from build123d import *

# Parameters (mm, degrees)
F0_W     = 326.6186
F0_H     = 45.9232
F0_W_2   = 5.842
F0_H_2   = 12.7
F1_DEPTH = 5.842
F2_R     = 3.175
F3_R     = 2.0828
F4_DEPTH = 25.4
F5_R     = 2.0828
F6_DEPTH = 25.4
F7_W     = 12.7
F7_H     = 5.842
F7_R     = 1.7526
F8_DEPTH = 25.4


with BuildPart() as f1:
    # F0 (on Front) → F1 (new body)
    with BuildSketch(Plane.XZ):
        Rectangle(F0_W, F0_H)
        with Locations((-157.2133, -12.7)):
            Rectangle(F0_W_2, F0_H_2, mode=Mode.SUBTRACT)
        with Locations((-134.3787, -12.7)):
            Rectangle(F0_W_2, F0_H_2, mode=Mode.SUBTRACT)
        with Locations((157.2133, -12.7)):
            Rectangle(F0_W_2, F0_H_2, mode=Mode.SUBTRACT)
        with Locations((-157.2133, 12.7)):
            Rectangle(F0_W_2, F0_H_2, mode=Mode.SUBTRACT)
        with Locations((-134.3787, 12.7)):
            Rectangle(F0_W_2, F0_H_2, mode=Mode.SUBTRACT)
        with Locations((157.2133, 12.7)):
            Rectangle(F0_W_2, F0_H_2, mode=Mode.SUBTRACT)
    extrude(amount=F1_DEPTH)

    # F2
    f2_edges = [f1.edges().sort_by_distance(p)[0] for p in [
        (-163.3093, -2.921, 22.9616),
        (-163.3093, -2.921, -22.9616),
        (163.3093, -2.921, 22.9616),
        (163.3093, -2.921, -22.9616),
    ]]
    fillet(f2_edges, radius=F2_R)

    # F3 (on face) → F4 (cut)
    with BuildSketch(Plane.XZ.offset(5.842)):
        with Locations((-134.3787, 0)):
            Circle(F3_R)
        with Locations((-157.2133, 0)):
            Circle(F3_R)
    extrude(amount=-F4_DEPTH, mode=Mode.SUBTRACT)

    # F5 (on face) → F6 (cut)
    with BuildSketch(Plane.XZ.offset(5.842)):
        with Locations((157.2133, 0)):
            Circle(F5_R)
    extrude(amount=-F6_DEPTH, mode=Mode.SUBTRACT)

    # F7 (on face) → F8 (cut)
    with BuildSketch(Plane.XZ.offset(5.842)):
        with Locations((-10.58418, 16.6116)):
            Rectangle(F7_W, F7_H)
        with Locations((27.51582, 16.6116)):
            Rectangle(F7_W, F7_H)
        with Locations((65.61582, 16.6116)):
            Rectangle(F7_W, F7_H)
        with Locations((8.46582, 16.6116)):
            Circle(F7_R)
        with Locations((46.56582, 16.6116)):
            Circle(F7_R)
        with Locations((-10.58418, -8.7884)):
            Rectangle(F7_W, F7_H)
        with Locations((27.51582, -8.7884)):
            Rectangle(F7_W, F7_H)
        with Locations((65.61582, -8.7884)):
            Rectangle(F7_W, F7_H)
        with Locations((8.46582, -8.7884)):
            Circle(F7_R)
        with Locations((46.56582, -8.7884)):
            Circle(F7_R)
    extrude(amount=-F8_DEPTH, mode=Mode.SUBTRACT)


solid = f1.part
Verification items for the finished model (mm, model axes). Give positions to 0.01 mm unless a question says otherwise; leave off trailing zeros. Write item = value, one per line.
(1) Draft check along X on faces 1 (the face through (-163.309, -3, 0)), 2 (the face through (163.309, -3, 0)), 3 (the face through (66, -3, 13.691)). Enter one of: released by +X, released by -X, zero draft, split by the parting line, or undercut.
Found:
face_1 = released by -X
face_2 = released by +X
face_3 = undercut
(2) Sectioned sample at A-A (y = -4.9). Give the number of separate pieces and of enclosed holes in the cut face, then the cut area to 3 significant figures.
Found:
separate_pieces = 1
enclosed_holes = 19
area = 14,000 mm2
(3) Material ranges on line 1 (Z direction, x = 65.5, y = -0.6); line 2 (X direction, y = -5.4, z = -17.5), recorded low to high.
Found:
line_1 = -22.96 to -11.71, -5.87 to 13.69, 19.53 to 22.96
line_2 = -163.31 to -160.13, -154.29 to -137.3, -131.46 to 154.29, 160.13 to 163.31
